```python
from build123d import *

# Parameters (mm, degrees)
MIRROREDSKETCH005_R = 2.15
PAD021_DEPTH        = 1.4
SKETCH093_R         = 0.7
SKETCH093_R_2       = 0.644462
SKETCH093_R_3       = 0.731859
POCKET013_DEPTH     = 1.401
PAD024_DEPTH        = 2


with BuildPart() as part:
    # MirroredSketch005 → Pad021 (new body)
    with BuildSketch(Plane.XY):
        with BuildLine():
            Line((0, 56.25), (0, 0.632))
            ThreePointArc((0, 0.632), (0.185109, 0.185109), (0.632, 0))
            Line((0.632, 0), (55.698332, 0))
            Line((55.698332, 0), (66.424272, -14.703544))
            Line((66.424272, -14.703544), (103.928425, -19.581139))
            Line((103.928425, -19.581139), (118.436579, -27.974316))
            ThreePointArc((118.436579, -27.974316), (119.477427, -28.111715), (120.309905, -27.472009))
            Line((120.309905, -27.472009), (133.73, -4.162))
            Line((133.73, -4.162), (133.73, 55.868))
            ThreePointArc((133.73, 55.868), (133.544891, 56.314891), (133.098, 56.5))
            Line((133.098, 56.5), (113.612, 56.5))
            ThreePointArc((112.98, 57.132), (113.165109, 56.685109), (113.612, 56.5))
            Line((112.98, 57.132), (112.98, 58.118))
            ThreePointArc((112.98, 58.118), (112.794891, 58.564891), (112.348, 58.75))
            Line((112.348, 58.75), (94.612, 58.75))
            ThreePointArc((93.98, 59.382), (94.165109, 58.935109), (94.612, 58.75))
            Line((93.98, 59.382), (93.98, 60.368))
            ThreePointArc((93.98, 60.368), (93.794891, 60.814891), (93.348, 61))
            Line((93.348, 61), (75.612, 61))
            ThreePointArc((74.98, 61.632), (75.165109, 61.185109), (75.612, 61))
            Line((74.98, 61.632), (74.98, 62.618))
            ThreePointArc((74.98, 62.618), (74.794891, 63.064891), (74.348, 63.25))
            Line((74.348, 63.25), (57.612, 63.25))
            ThreePointArc((57.612, 63.25), (57.165109, 63.064891), (56.98, 62.618))
            Line((56.98, 62.618), (56.98, 61.632))
            ThreePointArc((56.348, 61), (56.794891, 61.185109), (56.98, 61.632))
            Line((56.348, 61), (38.612, 61))
            ThreePointArc((38.612, 61), (38.165109, 60.814891), (37.98, 60.368))
            Line((37.98, 60.368), (37.98, 56.882))
            ThreePointArc((37.348, 56.25), (37.794891, 56.435109), (37.98, 56.882))
            Line((37.348, 56.25), (0, 56.25))
        make_face()
        with Locations((18.61, 37.509997)):
            Circle(MIRROREDSKETCH005_R, mode=Mode.SUBTRACT)
        with Locations((18.6, 18.76)):
            Circle(MIRROREDSKETCH005_R, mode=Mode.SUBTRACT)
        with Locations((108.3, -6.24)):
            Circle(MIRROREDSKETCH005_R, mode=Mode.SUBTRACT)
        with Locations((94.55, 41.5)):
            Circle(MIRROREDSKETCH005_R, mode=Mode.SUBTRACT)
        with Locations((61.84, 1.51)):
            Circle(MIRROREDSKETCH005_R, mode=Mode.SUBTRACT)
    extrude(amount=PAD021_DEPTH)

    # Sketch093 (on Face38 of Pad021) → Pocket013 (cut, through all)
    with BuildSketch(Plane.XY.offset(1.4)):
        with Locations((131.63, 53.8)):
            Circle(SKETCH093_R)
        with Locations((131.63, 51.7)):
            Circle(SKETCH093_R)
        with Locations((131.63, 49.6)):
            Circle(SKETCH093_R)
        with Locations((131.63, 47.5)):
            Circle(SKETCH093_R)
        with Locations((131.63, 45.4)):
            Circle(SKETCH093_R)
        with Locations((131.63, 43.3)):
            Circle(SKETCH093_R)
        with Locations((131.63, 41.2)):
            Circle(SKETCH093_R)
        with Locations((131.63, 39.1)):
            Circle(SKETCH093_R)
        with Locations((131.63, 37)):
            Circle(SKETCH093_R)
        with Locations((131.63, 34.9)):
            Circle(SKETCH093_R)
        with Locations((131.63, 32.8)):
            Circle(SKETCH093_R)
        with Locations((131.63, 30.7)):
            Circle(SKETCH093_R)
        with Locations((131.63, 28.6)):
            Circle(SKETCH093_R)
        with Locations((117.63, 53.8)):
            Circle(SKETCH093_R_2)
        with Locations((117.63, 51.7)):
            Circle(SKETCH093_R)
        with Locations((117.63, 49.6)):
            Circle(SKETCH093_R)
        with Locations((117.63, 47.5)):
            Circle(SKETCH093_R)
        with Locations((117.63, 45.4)):
            Circle(SKETCH093_R)
        with Locations((117.63, 43.3)):
            Circle(SKETCH093_R)
        with Locations((117.63, 41.2)):
            Circle(SKETCH093_R)
        with Locations((117.63, 39.1)):
            Circle(SKETCH093_R)
        with Locations((117.63, 37)):
            Circle(SKETCH093_R)
        with Locations((117.63, 34.868141)):
            Circle(SKETCH093_R_3)
        with Locations((117.63, 32.8)):
            Circle(SKETCH093_R)
        with Locations((117.63, 30.7)):
            Circle(SKETCH093_R)
        with Locations((117.63, 28.6)):
            Circle(SKETCH093_R)
    extrude(amount=-POCKET013_DEPTH, mode=Mode.SUBTRACT)

    # Sketch101 (on Face5 of Pocket013) → Pad024 (join)
    with BuildSketch(Plane.XY.offset(1.4)):
        Polygon((129.88, 24.6), (129.88, 18.6), (133.38, 18.6), (133.38, 24.6), (131.63, 24.6), align=None)
    extrude(amount=PAD024_DEPTH)


with BuildPart() as part_1:
    # Body005 placement: moved
    add(part.part.moved(Location((0, 0, 2))))


solid = part_1.part
```
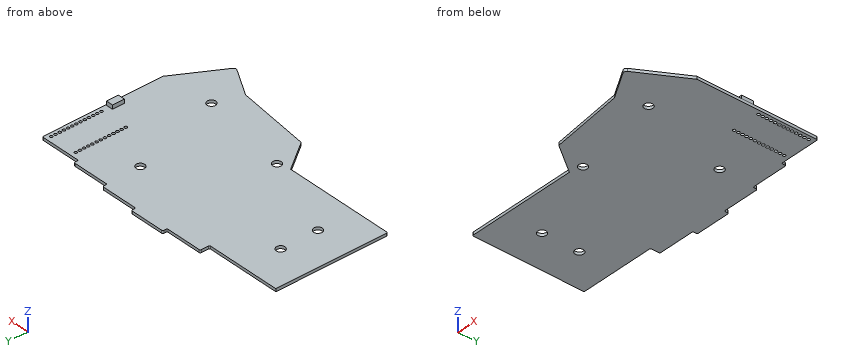
Geometry check sheet. Reference: the model listing, model coordinates, mm. Round coordinates to 2 decimals unless told otherwise and drop trailing zeros. Order: outer loops, then holes, each group sorted by start corner. A loop starts at its lowest first (then second) coordinate and runs counter-clockwise, first axis right, second up. Notation, with made-up numbers: (-2.5, -18.5) -> (15.5, -18.5) arc R27 cw to (15.5, 16.5) -> close; hole circle Ø10 at (75, -23). An arc over 180 degrees is marked (long way). Return JSON: item names as keys, results as strings. Group by question number.
Q1. Gauge pin test, flat ends, axial feed: pin 1 (2.5 mm diameter, centred on x = 18.61, y = 37.51, fed in from +Z); pin 2 (0.7 mm diameter, centred on x = 125.5, z = 2.5, fed in from +Y); pin 3 (1.5 mm diameter, centred on y = 59, z = 3, fed in from -X); pin 4 (2 mm diameter, centred on x = 131.63, y = 53.8, fed in from +Z). Record the tip position at first contact, or that the pin passes through.
Q2. Section check C-C, the plane x = 10. Record the boundary of the cut face in (y, z).
Q3. Material ranges on probe 1 along X at (y, z) = (49.6, 2.3); probe 2 along X at (y, z) = (30.5, 3.15); probe 3 along X at (y, z) = (37, 2.4), recorded low to high. Write a range as from..to.
Q4. Section check A-A, the plane y = -6.24. Record the boundary of the cut face in (x, z).
Q5. Section check B-B, the plane x = 108.3. Record the boundary of the cut face in (y, z).
Numbers:
{
 "1": {"pin 1": "through", "pin 2": "y = 56.5", "pin 3": "x = 37.98", "pin 4": "z = 3.4"},
 "2": {"outline": "(0, 2) -> (56.25, 2) -> (56.25, 3.4) -> (0, 3.4) -> close"},
 "3": {"probe 1": "0..116.93, 118.33..130.93, 132.33..133.73", "probe 2": "0..116.96, 118.3..130.96, 132.3..133.73", "probe 3": "0..16.52, 20.7..116.93, 118.33..130.93, 132.33..133.73"},
 "4": {"outline": "(60.25, 2) -> (106.15, 2) -> (106.15, 3.4) -> (60.25, 3.4) -> close; (110.45, 2) -> (132.53, 2) -> (132.53, 3.4) -> (110.45, 3.4) -> close"},
 "5": {"outline": "(-22.11, 2) -> (-8.39, 2) -> (-8.39, 3.4) -> (-22.11, 3.4) -> close; (-4.09, 2) -> (58.75, 2) -> (58.75, 3.4) -> (-4.09, 3.4) -> close"}
}
